Build history of the part. All positions in model axes, mm. Give positions to 0.01 mm unless a question says otherwise; leave off trailing zeros. Loops run counter-clockwise (first coordinate to the right, second up) from the corner with the lowest first, then second, coordinate; pieces in that order, holes last. Notation, with made-up numbers: M 19.5,-37 L 41.5,-37 A26 cw 41.5,-12 Z; hole C 89,43.25 d7. An arc over 180 degrees is marked long. Answer as a JSON object with one key per item and string values. Group by question number.
1. Drill centre lines: line 1 along Z through (x, y) = (350.5, 30); line 2 along Z through (x, y) = (252.5, 17); line 3 along Z through (x, y) = (83.5, 33.5). Where is each one in solid material? Low to high. Write a range as [from, to].
2. Slice it at D-D (z = 249). List the corners of the cut face in (x, y), then the cut area to 3 significant figures.
3. Slice it at A-A (y = 31). List the corners of the cut face in (x, z), then the cut area to 3 significant figures.
4. Slice it at B-B (z = -93). List the corners of the cut face in (x, y).
5. Drop flat-ended pins along their axis: pin 1 Ø1.5 at (x, y) = (-337, 5) entering from -Z; pin 2 Ø6 at (x, y) = (219.5, 11) entering from -Z; pin 3 Ø2 at (x, y) = (-93, 4) entering from +Z. Give the stop position or say it passes through.
6. Slice it at C-C (x = 175.5). List the corners of the cut face in (y, z), then the cut area to 3 significant figures.
from build123d import *

# Parameters (mm, degrees)
CROQUIS1_R              = 500
CROQUIS1_R_2            = 150
SALIENTE_EXTRUIR1_DEPTH = 40


with BuildPart() as part:
    # Croquis1 → Saliente-Extruir1 (new body)
    with BuildSketch(Plane(origin=(0, 0, 0), x_dir=(1, 0, 0), z_dir=(0, 1, 0))):
        with Locations(Location((0, 0, 0), (0, 0, 270))):
            Circle(CROQUIS1_R)
        with Locations(Location((0, 0, 0), (0, 0, 270))):
            Circle(CROQUIS1_R_2, mode=Mode.SUBTRACT)
        with BuildLine():
            ThreePointArc((-398.931865484, -230.323419925), (-184.304605999, 49.384270339), (-230.323419925, 398.931865484))
            ThreePointArc((-230.323419925, 398.931865484), (-444.95067941, 119.22417522), (-398.931865484, -230.323419925))
        make_face(mode=Mode.SUBTRACT)
        with BuildLine():
            ThreePointArc((398.931865484, -230.323419925), (49.384270339, -184.304605999), (-230.323419925, -398.931865484))
            ThreePointArc((-230.323419925, -398.931865484), (119.22417522, -444.95067941), (398.931865484, -230.323419925))
        make_face(mode=Mode.SUBTRACT)
        with BuildLine():
            ThreePointArc((0, 460.646839851), (134.92033566, 134.92033566), (460.646839851, 0))
            ThreePointArc((460.646839851, 0), (325.726504191, 325.726504191), (0, 460.646839851))
        make_face(mode=Mode.SUBTRACT)
    extrude(amount=SALIENTE_EXTRUIR1_DEPTH)


solid = part.part
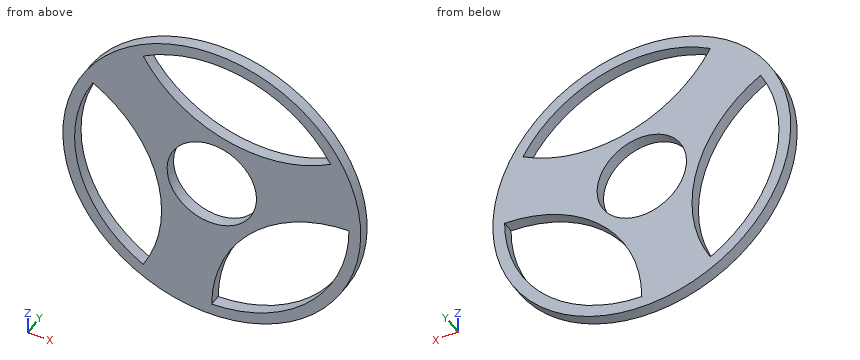
Established:
{
 "1": {"line 1": "z = [-356.58, -298.91], [-13.36, 206.04], [298.91, 356.58]", "line 2": "z = [-431.56, -385.28], [-49.71, 176.31], [385.28, 431.56]", "line 3": "z = [-492.98, -453.02], [-196.16, -124.61], [124.61, 176.54], [453.02, 492.98]"},
 "2": {"outline": "M -433.59,0 L -91.39,0 L -91.39,40 L -433.59,40 Z; M 387.55,0 L 433.59,0 L 433.59,40 L 387.55,40 Z", "area": "15,500 mm^2"},
 "3": {"outline": "C 0,0 d1000; hole M -398.93,230.32 A460.65 ccw -230.32,-398.93 A460.65 ccw Z; hole M -230.32,398.93 A460.65 ccw 398.93,230.32 A460.65 ccw Z; hole C 0,0 d300; hole M 0,-460.65 A460.65 ccw 460.65,0 A460.65 ccw Z", "area": "351,000 mm^2"},
 "4": {"outline": "M -491.27,0 L -451.16,0 L -451.16,40 L -491.27,40 Z; M -174.86,0 L -117.69,0 L -117.69,40 L -174.86,40 Z; M 117.69,0 L 183.1,0 L 183.1,40 L 117.69,40 Z; M 451.16,0 L 491.27,0 L 491.27,40 L 451.16,40 Z"},
 "5": {"pin 1": "stops at z = -370.05", "pin 2": "stops at z = -450.7", "pin 3": "stops at z = 491.46"},
 "6": {"outline": "M 0,-468.19 L 40,-468.19 L 40,-425.91 L 0,-425.91 Z; M 0,-98.86 L 40,-98.86 L 40,168.66 L 0,168.66 Z; M 0,425.91 L 40,425.91 L 40,468.19 L 0,468.19 Z", "area": "14,100 mm^2"}
}
